The listing builds one solid part. Answer for the finished solid, in the listing's coordinates (mm). Face numbers are marked on the shaded views. A direction names the side the tool comes from. Coordinates: 2 decimals unless noted, no trailing zeros. Order: outer loops, then holes, each group sorted by start corner. A loop starts at its lowest first (then second) coordinate and runs counter-clockwise, first axis right, second up. Notation, with made-up numbers: (84.5, 52) - (88.5, 52) arc R16 ccw to (88.5, 82) - close; hole circle Ø10 at (-19.75, -9.5). An arc over 180 degrees is marked (long way). Use a Markdown table: item, result. Add a question column.
Item 1: The part is cut by section A-A, the plane x = 6. Give the vertices of the cut face in (y, z), then the cut area to 3 significant figures.
Item 2: The part is cut by section B-B, the plane z = 76. Give the vertices of the cut face in (x, y).
Item 3: The part is cut by section D-D, the plane y = 9. Give the vertices of the cut face in (x, z).
Item 4: Flat-ended cylindrical pins translate along their axes: P1, Ø4, axis at x = 10.5, z = 49.5, coming from the +Y side; P2, Ø1.5, axis at x = 10, y = 3, coming from the +Z side. Find the tip coordinate at first contact, or state that the pin passes through.
Item 5: Find the intervals of material crossed by line 1 along Y through (x, z) = (6, 1.7); line 2 along X through (y, z) = (-5.75, 33); line 3 along Z through (x, y) = (-2, 0.5), in increasing order.
Item 6: The mould has two halves that part along X. Classify the marked faces 1, 2 and 3: released by +X, released by -X, zero draft, split by the parting line, or undercut.
Item 7: The part is cut by section C-C, the plane y = 5. Give the vertices of the cut face in (x, z).
Item 8: For the marked faces 4 and 5, determine the directions among +Z, -Z, +X, -X, +Y, -Y from which every point of the face is accessible in a straight line to the end or side of a thin tool.
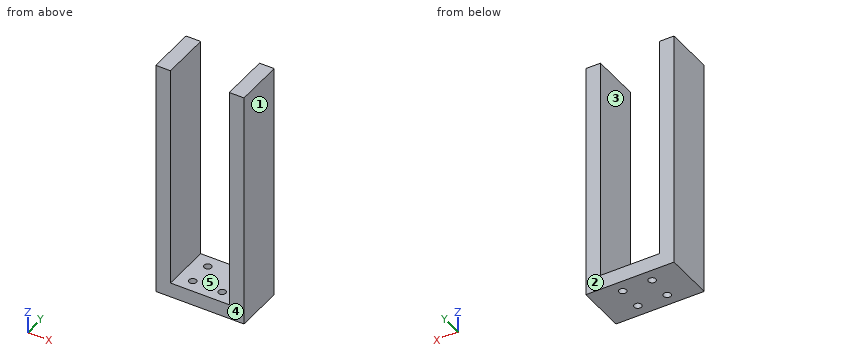
from build123d import *

# Parameters (mm, degrees)
SKETCH_1_W      = 6
SKETCH_1_H      = 20
SKETCH_1_W_2    = 24
SKETCH_1_R      = 1.5
EXTRUDE_1_DEPTH = 6
SKETCH_1_3_W    = 6
SKETCH_1_3_H    = 20
EXTRUDE_2_DEPTH = 98


with BuildPart() as part:
    # Sketch 1 → Extrude 1 (new body)
    # profile 1 of 3: a face of its own
    with BuildSketch(Plane.XY):
        with Locations((-15, 0)):
            Rectangle(SKETCH_1_W, SKETCH_1_H)
    # profile 2 of 3: a face of its own
    with BuildSketch(Plane.XY):
        Rectangle(SKETCH_1_W_2, SKETCH_1_H)
        with Locations((-6, -5)):
            Circle(SKETCH_1_R, mode=Mode.SUBTRACT)
        with Locations((6, -5)):
            Circle(SKETCH_1_R, mode=Mode.SUBTRACT)
        with Locations((-6, 5)):
            Circle(SKETCH_1_R, mode=Mode.SUBTRACT)
        with Locations((6, 5)):
            Circle(SKETCH_1_R, mode=Mode.SUBTRACT)
    # profile 3 of 3: a face of its own
    with BuildSketch(Plane.XY):
        with Locations((15, 0)):
            Rectangle(SKETCH_1_W, SKETCH_1_H)
    extrude(amount=EXTRUDE_1_DEPTH)

    # Sketch 1_3 → Extrude 2 (add)
    with BuildSketch(Plane.XY):
        with Locations((15, 0)):
            Rectangle(SKETCH_1_3_W, SKETCH_1_3_H)
        with Locations((-15, 0)):
            Rectangle(SKETCH_1_3_W, SKETCH_1_3_H)
    extrude(amount=EXTRUDE_2_DEPTH)


solid = part.part
Solution:
| question | item | result |
|---|---|---|
| 1 | outline | (-10, 0) - (-6.5, 0) - (-6.5, 6) - (-10, 6) - close; (-3.5, 0) - (3.5, 0) - (3.5, 6) - (-3.5, 6) - close; (6.5, 0) - (10, 0) - (10, 6) - (6.5, 6) - close |
| 1 | area | 84.0 mm2 |
| 2 | outline | (-18, -10) - (-12, -10) - (-12, 10) - (-18, 10) - close; (12, -10) - (18, -10) - (18, 10) - (12, 10) - close |
| 3 | outline | (-18, 0) - (18, 0) - (18, 98) - (12, 98) - (12, 6) - (-12, 6) - (-12, 98) - (-18, 98) - close |
| 4 | P1 | stops at y = 10 |
| 4 | P2 | stops at z = 6 |
| 5 | line 1 | y = -10 to -6.5, -3.5 to 3.5, 6.5 to 10 |
| 5 | line 2 | x = -18 to -12, 12 to 18 |
| 5 | line 3 | z = 0 to 6 |
| 6 | face 1 | released by +X |
| 6 | face 2 | zero draft |
| 6 | face 3 | undercut |
| 7 | outline | (-18, 0) - (-7.5, 0) - (-7.5, 6) - (-12, 6) - (-12, 98) - (-18, 98) - close; (-4.5, 0) - (4.5, 0) - (4.5, 6) - (-4.5, 6) - close; (7.5, 0) - (18, 0) - (18, 98) - (12, 98) - (12, 6) - (7.5, 6) - close |
| 8 | face 4 | +Z, -Z, +X, -X, -Y |
| 8 | face 5 | +Z, +Y, -Y |
